```python
from build123d import *

# Parameters (mm, degrees)
SKETCH1_R           = 3.925
BOSS_EXTRUDE1_DEPTH = 3.1
SKETCH2_R           = 1.49
CUT_EXTRUDE1_DEPTH  = 3.1
SKETCH3_R           = 1.49
BOSS_EXTRUDE2_DEPTH = 3


with BuildPart() as part:
    # Sketch1 → Boss-Extrude1 (new body)
    with BuildSketch(Plane(origin=(0, 0, 0), x_dir=(1, 0, 0), z_dir=(0, 1, 0))):
        with Locations(Location((0, 0, 0), (0, 0, 90))):
            Circle(SKETCH1_R)
    extrude(amount=BOSS_EXTRUDE1_DEPTH)

    # Sketch2 → Cut-Extrude1 (cut)
    with BuildSketch(Plane(origin=(0, 3.1, 0), x_dir=(1, 0, 0), z_dir=(0, 1, 0))):
        with Locations(Location((0, 0, 0), (0, 0, 270))):
            Circle(SKETCH2_R)
    extrude(amount=-CUT_EXTRUDE1_DEPTH, mode=Mode.SUBTRACT)

    # Sketch3 → Boss-Extrude2 (add)
    with BuildSketch(Plane(origin=(0, 3.1, 0), x_dir=(1, 0, 0), z_dir=(0, 1, 0))):
        with BuildLine():
            Line((-3.925, 0), (-3.925, -15))
            ThreePointArc((-3.925, -15), (-3.339213562, -16.414213562), (-1.925, -17))
            Line((-1.925, -17), (1.925, -17))
            ThreePointArc((1.925, -17), (3.339213562, -16.414213562), (3.925, -15))
            Line((3.925, -15), (3.925, 0))
            ThreePointArc((3.925, 0), (0, 3.925), (-3.925, 0))
        make_face()
        with Locations(Location((0, 0, 0), (0, 0, 270))):
            Circle(SKETCH3_R, mode=Mode.SUBTRACT)
    extrude(amount=BOSS_EXTRUDE2_DEPTH)


solid = part.part
```
For this review, take the finished solid that the model builds, in its own axes (mm). Give positions to 0.01 mm unless a question says otherwise; leave off trailing zeros. Order: outer loops, then holes, each group sorted by start corner. A loop starts at its lowest first (then second) coordinate and runs counter-clockwise, first axis right, second up.
1) Take a section at D-D (z = 3.5). Give the boundary of the cut face in (x, y) (3 decimals).
2) Take a section at C-C (y = 1.5). Give the boundary of the cut face in (x, z) (3 decimals), then the cut area to 3 significant figures.
3) The part is to be moulded in two halves that separate along Z. For faces 1 (the face through (-3.355, 4.579, 16.399)), 2 (the face through (1.477, 3.007, -0.194)), 3 (the face through (1.85, 3.69, -3.46)), say which applies: released by +Z, released by -Z, zero draft, split by the parting line, or undercut.
4) Take a section at A-A (x = 0). Give the boundary of the cut face in (y, z) (3 decimals), then the cut area to 3 significant figures.
5) Wall thickness on line 1 (X direction, y = 2, z = 0) (3 decimals); line 2 (Y direction, x = -3, z = 13.25); line 3 (Z direction, x = 0.75, y = 3): over which ranges is each line inside the solid? List them lowest first.
6) Take a section at B-B (z = -1.25). Give the boundary of the cut face in (x, y), then the cut area to 3 significant figures.
7) Insertion check: pin 1 (4 mm diameter, centred on x = -1.5, z = 7.5, fed in from -Y); pin 2 (3 mm diameter, centred on x = -2.5, y = 3, fed in from -Z). Each pin has a flat end and moves straight along its axis. Give the tip position at first contact, or say it passes through.
Derived:
1. outline: (-3.925, 3.1) - (-1.776, 3.1) - (-1.776, 0) - (1.776, 0) - (1.776, 3.1) - (3.925, 3.1) - (3.925, 6.1) - (-3.925, 6.1) - close
2. outline: circle Ø7.85 at (0, 0); hole circle Ø2.98 at (0, 0)
2. area: 41.4 mm2
3. face 1: released by +Z
3. face 2: undercut
3. face 3: split by the parting line
4. outline: (0, -3.925) - (6.1, -3.925) - (6.1, -1.49) - (0, -1.49) - close; (0, 1.49) - (6.1, 1.49) - (6.1, 17) - (3.1, 17) - (3.1, 3.925) - (0, 3.925) - close
4. area: 68.9 mm2
5. line 1: x = -3.925 to -1.49, 1.49 to 3.925
5. line 2: y = 3.1 to 6.1
5. line 3: z = -3.85 to -1.29, 1.29 to 3.85
6. outline: (-3.72, 0) - (-0.81, 0) - (-0.81, 6.1) - (-3.72, 6.1) - close; (0.81, 0) - (3.72, 0) - (3.72, 6.1) - (0.81, 6.1) - close
6. area: 35.5 mm2
7. pin 1: stops at y = 3.1
7. pin 2: stops at z = -3.8
